```python
from build123d import *

# Parameters (mm, degrees)
SCHIZZO2_R                    = 2.485
ESTRUSIONE_ESTRUSIONE1_DEPTH  = 68.1
TAGLIO_ESTRUSIONE1_DEPTH      = 69.19061849
TAGLIO_ESTRUSIONE1_DEPTH_BACK = 69.19061849
SCHIZZO3_W                    = 1.05
SCHIZZO3_H                    = 4.16


with BuildPart() as part:
    # Schizzo2 → Estrusione-Estrusione1 (new body)
    with BuildSketch(Plane(origin=(0, 0, 0), x_dir=(1, 0, 0), z_dir=(0, 1, 0))):
        with Locations(Location((0, 0, 0), (0, 0, 270))):
            Circle(SCHIZZO2_R)
    extrude(amount=ESTRUSIONE_ESTRUSIONE1_DEPTH)

    # Schizzo3 → Taglio-Estrusione1 (cut, two sides: drawn at the far end of the back side and taken through both)
    with BuildSketch(Plane.XY.offset(-TAGLIO_ESTRUSIONE1_DEPTH_BACK)):
        with Locations((-1.96, 65.23)):
            Rectangle(SCHIZZO3_W, SCHIZZO3_H)
        with Locations((-1.96, 2.87)):
            Rectangle(SCHIZZO3_W, SCHIZZO3_H)
    extrude(amount=TAGLIO_ESTRUSIONE1_DEPTH + TAGLIO_ESTRUSIONE1_DEPTH_BACK, mode=Mode.SUBTRACT)


solid = part.part
```
Could you check a few things on this model? Use its own coordinates, in mm. A direction names the side the tool comes from. Round coordinates to 2 decimals unless told otherwise and drop trailing zeros. Loops run counter-clockwise (first coordinate to the right, second up) from the corner with the lowest first, then second, coordinate; pieces in that order, holes last. Notation, with made-up numbers: (-10.75, 42) - (-4.75, 42) arc R11 cw to (-4.75, 58) - close; hole circle Ø8 at (61.25, 42). An arc over 180 degrees is marked (long way). Answer in a Markdown table with one row per item. Add a question column.
(1) If we section it at C-C (x = 1.6): Please give me the cut outline in (y, z), plus the area to 3 significant figures.
(2) I need wall thicknesses on line 1 along X through (y, z) = (59, -1.45); line 2 along X through (y, z) = (22, -0.1); line 3 along Z through (x, y) = (-0.5, 29). Which ranges of each line are inside material? Lowest first, please.
(3) I'm going to push a flat-ended pin straight in: pin 1 (1 mm diameter, centred on y = 43.5, z = 1.5, fed in from +X). Where does the tip first touch, or does it pass through?
(4) If we section it at B-B (y = 40.5): Please give me the cut outline in (x, z) (3 decimals).
(5) If we section it at A-A (z = 0): Please give me the cut outline in (x, y) (3 decimals), plus the area to 3 significant figures.
(6) For faces 1 (the face through (0, 68.1, 0)), 2 (the face through (-1.435, 65, 0)), which set-ups out of +Z, -Z, +X, -X, +Y, -Y let a thin tool reach every point of the face, with its end or its side?
Model answer:
| question | item | result |
|---|---|---|
| 1 | outline | (0, -1.9) - (68.1, -1.9) - (68.1, 1.9) - (0, 1.9) - close |
| 1 | area | 259 mm² |
| 2 | line 1 | x = -2.02 to 2.02 |
| 2 | line 2 | x = -2.48 to 2.48 |
| 2 | line 3 | z = -2.43 to 2.43 |
| 3 | pin 1 | stops at x = 2.27 |
| 4 | outline | circle Ø4.97 at (0, 0) |
| 5 | outline | (-2.485, 0) - (2.485, 0) - (2.485, 68.1) - (-2.485, 68.1) - (-2.485, 67.31) - (-1.435, 67.31) - (-1.435, 63.15) - (-2.485, 63.15) - (-2.485, 4.95) - (-1.435, 4.95) - (-1.435, 0.79) - (-2.485, 0.79) - close |
| 5 | area | 330 mm² |
| 6 | face 1 | +Z, -Z, +X, -X, +Y |
| 6 | face 2 | +Z, -Z, -X |
